Work out the finished part from the listing and answer in its coordinate system (mm). Face numbers are marked on the shaded views. A direction names the side the tool comes from. Coordinates: 2 decimals unless noted, no trailing zeros. Loops run counter-clockwise (first coordinate to the right, second up) from the corner with the lowest first, then second, coordinate; pieces in that order, holes last. Notation, with made-up numbers: (-17.75, -17) - (25.25, -17) arc R17 ccw to (25.25, 11) - close; hole circle Ø8 at (50, 29). An arc over 180 degrees is marked (long way). Write each question's results on one line, items separated by ' | '. Start each with the question number.
Item 1: A tool of negligible diameter and unlimited length cuts with its end or side. For the marked faces 5 and 6, from which of +Z, -Z, +X, -X, +Y, -Y can it reach the whole face along a straight path? Write none if from no direction.
Item 2: This flat-tipped pin is pushed along its axis until it touches: pin 1 Ø5 at (y, z) = (5, -1.5) entering from +X. Where does it stop, or does it pass through?
Item 3: For a pull along Y with two mould halves and no side action, classify the marked faces 1, 2, 3 and 4 as +Y half, -Y half, draft (parallel to the pull), parting line (faces both ways), or undercut.
Item 4: Consider probe 1 along Z at (x, y) = (3.5, 3.5); probe 2 along Y at (x, z) = (3.5, -1.5); probe 3 along X at (y, z) = (4.5, -2). Determine where each line is inside the solid, lowest interval first. Write a range as [from, to].
Item 5: Section B-B, the plane y = 3.75 is taken. Write down the section's boundary in (x, z), plus the area to 3 significant figures.
Item 6: Section A-A, the plane z = -3.25 is taken. Write down the section's boundary in (x, y).
from build123d import *

# Parameters (mm, degrees)
BOSS_EXTRUDE1_DEPTH      = 5
BOSS_EXTRUDE1_DEPTH_BACK = 5
SKETCH1_W                = 10
SKETCH1_H                = 15
SKETCH3_W                = 9
SKETCH3_H                = 6
CUT_EXTRUDE2_DEPTH       = 2


with BuildPart() as part:
    # Sketch1 → Boss-Extrude1 (new, two sides: drawn at the far end of the back side and taken through both)
    with BuildSketch(Plane.XY.offset(-BOSS_EXTRUDE1_DEPTH_BACK)):
        with Locations((0, 1.32209169)):
            Rectangle(SKETCH1_W, SKETCH1_H)
    extrude(amount=BOSS_EXTRUDE1_DEPTH + BOSS_EXTRUDE1_DEPTH_BACK)

    # Sketch3 → Cut-Extrude2 (cut)
    with BuildSketch(Plane(origin=(5, 0, 0), x_dir=(0, 0, -1), z_dir=(1, 0, 0))):
        with Locations((0, 5.32209169)):
            Rectangle(SKETCH3_W, SKETCH3_H)
    extrude(amount=-CUT_EXTRUDE2_DEPTH, mode=Mode.SUBTRACT)


solid = part.part
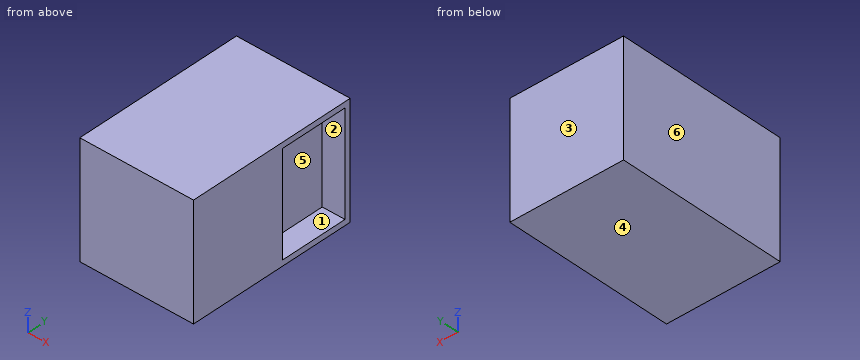
Answer key:
1) face 5: +X | face 6: +Z, -Z, -X, +Y, -Y
2) pin 1: stops at x = 3
3) face 1: undercut | face 2: undercut | face 3: +Y half | face 4: draft
4) probe 1: z = [-5, -4.5], [4.5, 5] | probe 2: y = [-6.18, 2.32], [8.32, 8.82] | probe 3: x = [-5, 3]
5) outline: (-5, -5) - (5, -5) - (5, -4.5) - (3, -4.5) - (3, 4.5) - (5, 4.5) - (5, 5) - (-5, 5) - close | area: 82.0 mm^2
6) outline: (-5, -6.18) - (5, -6.18) - (5, 2.32) - (3, 2.32) - (3, 8.32) - (5, 8.32) - (5, 8.82) - (-5, 8.82) - close
